from build123d import *

# Parameters (mm, degrees)
BOSS_EXTRU_1_DEPTH                  = 26
ESQUISSE2_W                         = 42.1
ESQUISSE2_H                         = 42.3
BOSS_EXTRU_2_DEPTH                  = 11
ESQUISSE3_W                         = 11
ESQUISSE3_H                         = 42.3
BOSS_EXTRU_3_DEPTH                  = 0.2
ESQUISSE4_W                         = 42.3
ESQUISSE4_H                         = 42.3
BOSS_EXTRU_4_DEPTH                  = 11
ESQUISSE5_R                         = 11
BOSS_EXTRU_5_DEPTH                  = 2
DIAM_TRE_DU_PER_AGE_9_0_9_1_D       = 9
DIAM_TRE_DU_PER_AGE_9_0_9_1_DEPTH   = 2
ESQUISSE8_R                         = 2.5
BOSS_EXTRU_6_DEPTH                  = 24.5
ENL_V_START                         = -15
ENL_V_MAT_EXTRU_1_DEPTH             = 15
DIAM_TRE_DU_PER_AGE_2_5_2_5_1_D     = 2.5
DIAM_TRE_DU_PER_AGE_2_5_2_5_1_DEPTH = 7.5
DIAM_TRE_DU_PER_AGE_2_5_2_5_1_TIP   = 0.751075774
DIAM_TRE_DU_PER_AGE_4_0_4_1_D       = 4
DIAM_TRE_DU_PER_AGE_4_0_4_1_DEPTH   = 2
DIAM_TRE_DU_PER_AGE_10_0_10_1_D     = 10
DIAM_TRE_DU_PER_AGE_10_0_10_1_DEPTH = 2
CHANFREIN1_SIZE                     = 4
CONG_1_R                            = 0.2


with BuildPart() as part:
    # Esquisse1 → Boss.-Extru.1 (new body)
    with BuildSketch(Plane.XY.offset(-11)):
        Polygon((20.95, 15.95), (15.95, 20.95), (-15.95, 20.95), (-20.95, 15.95), (-20.95, -15.95), (-15.95, -20.95), (15.95, -20.95), (20.95, -15.95), align=None)
    extrude(amount=-BOSS_EXTRU_1_DEPTH)

    # Esquisse2 → Boss.-Extru.2 (add)
    with BuildSketch(Plane(origin=(0, 0, -37), x_dir=(-1, 0, 0), z_dir=(0, 0, -1))):
        with Locations((-0.1, 0)):
            Rectangle(ESQUISSE2_W, ESQUISSE2_H)
    extrude(amount=BOSS_EXTRU_2_DEPTH)

    # Esquisse3 → Boss.-Extru.3 (add)
    with BuildSketch(Plane.ZY.offset(20.95)):
        with Locations((-34.5, 0)):
            Rectangle(ESQUISSE3_W, ESQUISSE3_H)
    extrude(amount=BOSS_EXTRU_3_DEPTH)

    # Esquisse4 → Boss.-Extru.4 (add)
    with BuildSketch(Plane(origin=(0, 0, -11), x_dir=(-1, 0, 0), z_dir=(0, 0, -1))):
        Rectangle(ESQUISSE4_W, ESQUISSE4_H)
    extrude(amount=-BOSS_EXTRU_4_DEPTH)

    # Esquisse5 → Boss.-Extru.5 (add)
    with BuildSketch(Plane.XY):
        with Locations(Location((0, 0, 0), (0, 0, 180))):
            Circle(ESQUISSE5_R)
    extrude(amount=BOSS_EXTRU_5_DEPTH)

    # Diamètre du perçage Ø9.0 (9)1
    with Locations(Plane.XY.offset(2)):
        with Locations((0, 0)):
            Hole(DIAM_TRE_DU_PER_AGE_9_0_9_1_D / 2, depth=DIAM_TRE_DU_PER_AGE_9_0_9_1_DEPTH)

    # Esquisse8 → Boss.-Extru.6 (add)
    with BuildSketch(Plane.XY):
        with Locations(Location((0, 0, 0), (0, 0, 180))):
            Circle(ESQUISSE8_R)
    extrude(amount=BOSS_EXTRU_6_DEPTH)

    # Esquisse9 → Enlèv. mat.-Extru.1 (cut)
    with BuildSketch(Plane.XY.offset(24.5).offset(ENL_V_START)):
        with BuildLine():
            Line((1.5, -2), (-1.5, -2))
            ThreePointArc((-1.5, -2), (0, -2.5), (1.5, -2))
        make_face()
    extrude(amount=ENL_V_MAT_EXTRU_1_DEPTH, mode=Mode.SUBTRACT)

    # Diamètre du perçage Ø2.5 (2.5)1
    with Locations(Plane.XY):
        with Locations((-15.5, 15.5), (-15.5, -15.5), (15.5, -15.5), (15.5, 15.5)):
            Hole(DIAM_TRE_DU_PER_AGE_2_5_2_5_1_D / 2, depth=DIAM_TRE_DU_PER_AGE_2_5_2_5_1_DEPTH)
            with Locations((0, 0, -(DIAM_TRE_DU_PER_AGE_2_5_2_5_1_DEPTH + DIAM_TRE_DU_PER_AGE_2_5_2_5_1_TIP / 2))):  # 118° drill point
                Cone(0, DIAM_TRE_DU_PER_AGE_2_5_2_5_1_D / 2, DIAM_TRE_DU_PER_AGE_2_5_2_5_1_TIP, mode=Mode.SUBTRACT)

    # Diamètre du perçage Ø4.0 (4)1
    with Locations(Plane(origin=(0, 0, -48), x_dir=(-1, 0, 0), z_dir=(0, 0, -1))):
        with Locations((-15.5, -15.5), (-15.5, 15.5), (15.5, 15.5), (15.5, -15.5)):
            Hole(DIAM_TRE_DU_PER_AGE_4_0_4_1_D / 2, depth=DIAM_TRE_DU_PER_AGE_4_0_4_1_DEPTH)

    # Diamètre du perçage Ø10.0 (10)1
    with Locations(Plane(origin=(0, 0, -48), x_dir=(-1, 0, 0), z_dir=(0, 0, -1))):
        with Locations((0, 0)):
            Hole(DIAM_TRE_DU_PER_AGE_10_0_10_1_D / 2, depth=DIAM_TRE_DU_PER_AGE_10_0_10_1_DEPTH)

    # Chanfrein1
    chanfrein1_edges = [part.edges().sort_by_distance(p)[0] for p in [
        (21.15, 21.15, -42.5),
        (-21.15, -21.15, -34.5),
        (21.15, -21.15, -42.5),
        (-21.15, 21.15, -5.5),
        (-21.15, -21.15, -5.5),
        (21.15, -21.15, -5.5),
        (-21.15, 21.15, -34.5),
        (21.15, 21.15, -5.5),
    ]]
    chamfer(chanfrein1_edges, length=CHANFREIN1_SIZE)

    # Congé1
    cong_1_edges = [part.edges().sort_by_distance(p)[0] for p in [
        (20.95, -15.95, -24),
        (15.95, -20.95, -24),
        (-15.95, -20.95, -24),
        (-15.95, 20.95, -24),
        (15.95, 20.95, -24),
        (20.95, 15.95, -24),
        (-20.95, 15.95, -20),
        (-20.95, -15.95, -20),
    ]]
    fillet(cong_1_edges, radius=CONG_1_R)


solid = part.part
Work out the finished part from the listing and answer in its coordinate system (mm). A direction names the side the tool comes from. Coordinates: 2 decimals unless noted, no trailing zeros. Write each loop counter-clockwise with the first axis right and the second up, starting at its lowest first coordinate (ties: lowest second). Pieces come first, ordered by that corner, then holes. Notation, with made-up numbers: M 21.5,39.5 L 48.5,39.5 A16 cw 48.5,58.5 Z; hole C -33,-35.75 d3. An arc over 180 degrees is marked long. Use one line per item in the form item = value. Start each with the question number.
1. The part is cut by section D-D (z = 18.5). Give the vertices of the cut face in (x, y).
2. The part is cut by section B-B (z = -25). Give the vertices of the cut face in (x, y).
3. Straight lines are drawn through the part: probe 1 along X at (y, z) = (-15.5, -2.5); probe 2 along Y at (x, z) = (0, -46.5); probe 3 along Z at (x, y) = (-8.5, 15). For each, find the intervals that lie inside material, in ascending order. Write a range as from..to.
4. A tool of negligible diameter and unlimited length cuts with its end or side. For faces 1 (the face through (19, 19, -37)), 2 (the face through (-16, -15, -46)), 3 (the face through (0, 21.15, -6)), 4 (the face through (0.59, 4.46, 0.99)), from which of +Z, -Z, +X, -X, +Y, -Y can it reach the whole face along a straight path? Write none if from no direction.
5. The mould has two halves that part along Y. Classify faces 5 (the face through (-20.95, 0, -44)), 6 (the face through (-16, 16, -46)), 7 (the face through (-19.2, 19.1, -5.6)), 8 (the face through (18.4, -18.5, -23.8)): released by +Y, released by -Y, zero draft, split by the parting line, or undercut.
6. Each of these flat-tipped pins is pushed along its axis until it touches: P1, Ø10, axis at x = 11.5, z = 2, coming from the -Y side; P2, Ø4, axis at y = 4, z = -45.5, coming from the -X side; P3, Ø3, axis at x = 15.5, y = -15.5, coming from the +Z side; P4, Ø10, axis at x = 2, y = -11.5, coming from the +Z side. Where does it stop, or does it pass through?
7. The part is cut by section C-C (y = 7). Give the vertices of the cut face in (x, z).
Evaluation:
q1.outline = M -1.5,-2 L 1.5,-2 A2.5 ccw long Z
q2.outline = M -20.95,-15.87 A0.2 ccw -20.89,-16.01 L -16.01,-20.89 A0.2 ccw -15.87,-20.95 L 15.87,-20.95 A0.2 ccw 16.01,-20.89 L 20.89,-16.01 A0.2 ccw 20.95,-15.87 L 20.95,15.87 A0.2 ccw 20.89,16.01 L 16.01,20.89 A0.2 ccw 15.87,20.95 L -15.87,20.95 A0.2 ccw -16.01,20.89 L -20.89,16.01 A0.2 ccw -20.95,15.87 Z
q3.probe_1 = -21.15..-16.75, -14.25..14.25, 16.75..21.15
q3.probe_2 = -21.15..-5, 5..21.15
q3.probe_3 = -48..0
q4.face_1 = none
q4.face_2 = -Z
q4.face_3 = +Z, -Z, +X, -X, +Y
q4.face_4 = +Z
q5.face_5 = zero draft
q5.face_6 = undercut
q5.face_7 = released by +Y
q5.face_8 = released by -Y
q6.P1 = -21.15
q6.P2 = -20.95
q6.P3 = 0
q6.P4 = 2
q7.outline = M -21.15,-40 L -20.95,-40 L -20.95,-48 L 21.15,-48 L 21.15,-37 L 20.95,-37 L 20.95,-11 L 21.15,-11 L 21.15,0 L 8.49,0 L 8.49,2 L -8.49,2 L -8.49,0 L -21.15,0 L -21.15,-11 L -20.95,-11 L -20.95,-29 L -21.15,-29 Z
